from build123d import *

# Parameters (mm, degrees)
SKETCH1_W           = 85
SKETCH1_H           = 65
SKETCH1_R           = 1.81
SKETCH1_W_2         = 14.5
SKETCH1_H_2         = 4.1
SKETCH1_W_3         = 9.8
SKETCH1_H_3         = 3.74
SKETCH1_W_4         = 10.3
SKETCH1_H_4         = 5.05
SKETCH1_W_5         = 73.7
SKETCH1_H_5         = 1.2
SKETCH1_W_6         = 45.6
SKETCH1_H_6         = 2.7
SKETCH1_W_7         = 41.8
BOSS_EXTRUDE1_DEPTH = 6
FILLET1_R           = 3


with BuildPart() as part:
    # Sketch1 → Boss-Extrude1 (new body)
    with BuildSketch(Plane(origin=(0, 0, 0), x_dir=(1, 0, 0), z_dir=(0, 1, 0))):
        Rectangle(SKETCH1_W, SKETCH1_H)
        with Locations((32.67, 5.206342289)):
            Circle(SKETCH1_R, mode=Mode.SUBTRACT)
        Polygon((37.5, -23.359842136), (27.84, -23.359842136), (27.84, -17.909842136), (30.61, -17.909842136), (30.61, -9.109842136), (34.73, -9.109842136), (34.73, -17.909842136), (37.5, -17.909842136), align=None, mode=Mode.SUBTRACT)
        with BuildLine():
            Line((23.3025, -23.359842136), (9.9325, -23.359842136))
            Line((9.9325, -23.359842136), (9.9325, -19.369842136))
            Line((9.9325, -19.369842136), (12.5525, -19.369842136))
            Line((12.5525, -19.369842136), (12.5525, -5.394842136))
            ThreePointArc((12.5525, -5.394842136), (16.6175, -1.329842136), (20.6825, -5.394842136))
            Line((20.6825, -5.394842136), (20.6825, -19.369842136))
            Line((20.6825, -19.369842136), (23.3025, -19.369842136))
            Line((23.3025, -19.369842136), (23.3025, -23.359842136))
        make_face(mode=Mode.SUBTRACT)
        with Locations((-2.165, -21.309842136)):
            Rectangle(SKETCH1_W_2, SKETCH1_H_2, mode=Mode.SUBTRACT)
        with Locations((-18.4625, -21.489842136)):
            Rectangle(SKETCH1_W_3, SKETCH1_H_3, mode=Mode.SUBTRACT)
        with Locations((-32.35, -20.834842136)):
            Rectangle(SKETCH1_W_4, SKETCH1_H_4, mode=Mode.SUBTRACT)
        with Locations((0, 28.473253228)):
            Rectangle(SKETCH1_W_5, SKETCH1_H_5, mode=Mode.SUBTRACT)
        with Locations((14.05, 23.086178608)):
            Rectangle(SKETCH1_W_6, SKETCH1_H_6, mode=Mode.SUBTRACT)
        with Locations((15.95, 16.43449293)):
            Rectangle(SKETCH1_W_7, SKETCH1_H_6, mode=Mode.SUBTRACT)
    extrude(amount=BOSS_EXTRUDE1_DEPTH)

    # Fillet1
    fillet1_edges = [part.edges().sort_by_distance(p)[0] for p in [
        (42.5, 3, 32.5),
        (-42.5, 3, 32.5),
        (-42.5, 3, -32.5),
        (42.5, 3, -32.5),
    ]]
    fillet(fillet1_edges, radius=FILLET1_R)


solid = part.part
Can you work these out from the model? Positions are in its coordinate system, mm. A direction names the side the tool comes from. Coordinates: 2 decimals unless noted, no trailing zeros. Order: outer loops, then holes, each group sorted by start corner. A loop starts at its lowest first (then second) coordinate and runs counter-clockwise, first axis right, second up. Notation, with made-up numbers: (57.25, 45.5) -> (100.25, 45.5) arc R27 ccw to (100.25, 80.5) -> close; hole circle Ø5 at (-25, -10.5). An arc over 180 degrees is marked (long way). Use one line per item in the form item = value.
Q1. Which directions (+Z, -Z, +X, -X, +Y, -Y) give clear straight access to the entire face, cutting with the end or side of a thin tool? Please do faces 4 (the face through (16, 3, -15.084)), 5 (the face through (-41.64, 3.04, 31.6)).
From the geometry:
face_4 = +Y, -Y
face_5 = +Z, -X, +Y, -Y
Q2. Imagine slicing it at A-A, the plane z = 16.5. List the corners of the cut face in (x, y) for me, then the cut area to 4 significant figures.
From the geometry:
outline = (-42.5, 0) -> (12.55, 0) -> (12.55, 6) -> (-42.5, 6) -> close; (20.68, 0) -> (30.61, 0) -> (30.61, 6) -> (20.68, 6) -> close; (34.73, 0) -> (42.5, 0) -> (42.5, 6) -> (34.73, 6) -> close
area = 436.5 mm²
Q3. I need wall thicknesses on L1, parallel to X at y = 3.7, z = 11; L2, parallel to Z at x = 32.67, y = 2.55; L3, parallel to Z at x = 12, y = 2.7. Which ranges of each line are inside material? Lowest first, please.
From the geometry:
L1 = -42.5 to 12.55, 20.68 to 30.61, 34.73 to 42.5
L2 = -32.5 to -29.07, -27.87 to -24.44, -21.74 to -17.78, -15.08 to -7.02, -3.4 to 9.11, 23.36 to 32.5
L3 = -32.5 to -29.07, -27.87 to -24.44, -21.74 to -17.78, -15.08 to 19.37, 23.36 to 32.5
Q4. Imagine slicing it at B-B, the plane x = -17. List the corners of the cut face in (y, z) for me.
From the geometry:
outline = (0, -32.5) -> (6, -32.5) -> (6, -29.07) -> (0, -29.07) -> close; (0, -27.87) -> (6, -27.87) -> (6, 19.62) -> (0, 19.62) -> close; (0, 23.36) -> (6, 23.36) -> (6, 32.5) -> (0, 32.5) -> close
Q5. Imagine slicing it at D-D, the plane x = 16. List the corners of the cut face in (y, z) for me.
From the geometry:
outline = (0, -32.5) -> (6, -32.5) -> (6, -29.07) -> (0, -29.07) -> close; (0, -27.87) -> (6, -27.87) -> (6, -24.44) -> (0, -24.44) -> close; (0, -21.74) -> (6, -21.74) -> (6, -17.78) -> (0, -17.78) -> close; (0, -15.08) -> (6, -15.08) -> (6, 1.38) -> (0, 1.38) -> close; (0, 23.36) -> (6, 23.36) -> (6, 32.5) -> (0, 32.5) -> close
Q6. We'd pull the mould along Z, two halves only. Please class faces 1 (the face through (-19, 3, 19.62)), 2 (the face through (-1, 6, 0)), 3 (the face through (-1, 3, 32.5)): released by +Z, released by -Z, zero draft, split by the parting line, or undercut.
From the geometry:
face_1 = undercut
face_2 = zero draft
face_3 = released by +Z
Q7. Imagine slicing it at C-C, the plane x = 32.67. List the corners of the cut face in (y, z) for me, then the cut area to 3 significant figures.
From the geometry:
outline = (0, -32.5) -> (6, -32.5) -> (6, -29.07) -> (0, -29.07) -> close; (0, -27.87) -> (6, -27.87) -> (6, -24.44) -> (0, -24.44) -> close; (0, -21.74) -> (6, -21.74) -> (6, -17.78) -> (0, -17.78) -> close; (0, -15.08) -> (6, -15.08) -> (6, -7.02) -> (0, -7.02) -> close; (0, -3.4) -> (6, -3.4) -> (6, 9.11) -> (0, 9.11) -> close; (0, 23.36) -> (6, 23.36) -> (6, 32.5) -> (0, 32.5) -> close
area = 243 mm²
